Can you work these out from the model? Positions are in its coordinate system, mm. A direction names the side the tool comes from. Give positions to 0.01 mm unless a question says otherwise; leave off trailing zeros. Loops run counter-clockwise (first coordinate to the right, second up) from the corner with the lowest first, then second, coordinate; pieces in that order, holes last.
from build123d import *

# Parameters (mm, degrees)
SKETCH1_W           = 21
SKETCH1_H           = 10.7
SKETCH1_W_2         = 18
SKETCH1_H_2         = 7.7
BOSS_EXTRUDE1_DEPTH = 6
FILLET1_R           = 0.6
FILLET2_R           = 1.7


with BuildPart() as part:
    # Sketch1 → Boss-Extrude1 (new body)
    with BuildSketch(Plane(origin=(0, 0, 0), x_dir=(0, 0, -1), z_dir=(1, 0, 0))):
        Rectangle(SKETCH1_W, SKETCH1_H)
        Rectangle(SKETCH1_W_2, SKETCH1_H_2, mode=Mode.SUBTRACT)
    extrude(amount=BOSS_EXTRUDE1_DEPTH)

    # Fillet1
    fillet1_edges = [part.edges().sort_by_distance(p)[0] for p in [
        (3, -3.85, -9),
        (3, 3.85, -9),
        (3, 3.85, 9),
        (3, -3.85, 9),
    ]]
    fillet(fillet1_edges, radius=FILLET1_R)

    # Fillet2
    fillet2_edges = [part.edges().sort_by_distance(p)[0] for p in [
        (3, -5.35, -10.5),
        (3, -5.35, 10.5),
        (3, 5.35, 10.5),
        (3, 5.35, -10.5),
    ]]
    fillet(fillet2_edges, radius=FILLET2_R)


solid = part.part
(1) Suppose I cut it at C-C on x = 1.2. List the corners of the cut face in (y, z) for me, plus the area to 3 significant figures.
Returned:
outline: (-5.35, -8.8) arc R1.7 ccw to (-3.65, -10.5) - (3.65, -10.5) arc R1.7 ccw to (5.35, -8.8) - (5.35, 8.8) arc R1.7 ccw to (3.65, 10.5) - (-3.65, 10.5) arc R1.7 ccw to (-5.35, 8.8) - close; hole (-3.85, -8.4) arc R0.6 ccw to (-3.25, -9) - (3.25, -9) arc R0.6 ccw to (3.85, -8.4) - (3.85, 8.4) arc R0.6 ccw to (3.25, 9) - (-3.25, 9) arc R0.6 ccw to (-3.85, 8.4) - close
area: 83.9 mm2
(2) Which directions (+Z, -Z, +X, -X, +Y, -Y) give clear straight access to the entire face, cutting with the end or side of a thin tool? Please do faces 1 (the flat face through (6, -5, 0)), 2 (the flat face through (3, 0, 9)).
Returned:
face 1: +Z, -Z, +X, +Y, -Y
face 2: +X, -X
(3) Suppose I cut it at B-B on z = 7. List the corners of the cut face in (x, y) for me.
Returned:
outline: (0, -5.35) - (6, -5.35) - (6, -3.85) - (0, -3.85) - close; (0, 3.85) - (6, 3.85) - (6, 5.35) - (0, 5.35) - close
(4) Please list where these lines run through material, in increasing order: probe 1 along Z at (x, y) = (2.6, 3.25); probe 2 along Y at (x, z) = (4.3, -5.5); probe 3 along Y at (x, z) = (1.25, -8.75).
Returned:
probe 1: z = -10.5 to -9, 9 to 10.5
probe 2: y = -5.35 to -3.85, 3.85 to 5.35
probe 3: y = -5.35 to -3.74, 3.74 to 5.35
(5) Suppose I cut it at A-A on y = -1.75. List the corners of the cut face in (x, z) for me.
Returned:
outline: (0, -10.5) - (6, -10.5) - (6, -9) - (0, -9) - close; (0, 9) - (6, 9) - (6, 10.5) - (0, 10.5) - close
